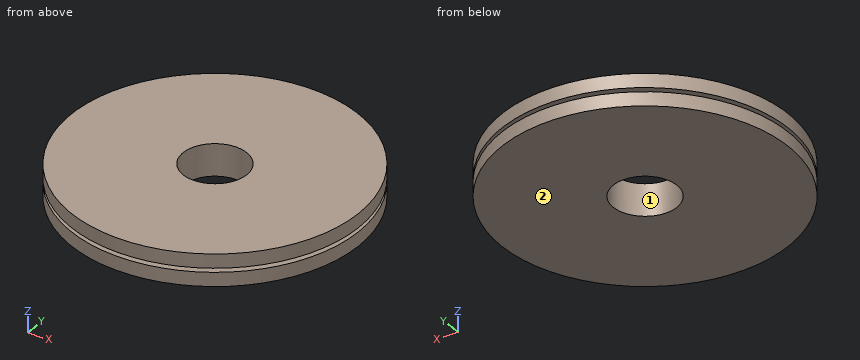
```python
from build123d import *

# Parameters (mm, degrees)
SKETCH1_R           = 57.15
SKETCH1_R_2         = 12.7
BOSS_EXTRUDE1_DEPTH = 12.7
SKETCH3_R           = 57.15
SKETCH3_R_2         = 53.975
CUT_EXTRUDE1_DEPTH  = 0.8001


with BuildPart() as part:
    # Sketch1 → Boss-Extrude1 (new body)
    with BuildSketch(Plane.XY):
        Circle(SKETCH1_R)
        Circle(SKETCH1_R_2, mode=Mode.SUBTRACT)
    extrude(amount=BOSS_EXTRUDE1_DEPTH)

    # Sketch3 → Cut-Extrude1 (cut, symmetric)
    with BuildSketch(Plane(origin=(0, 0, 6.35), x_dir=(-1, 0, 0), z_dir=(0, 0, -1))):
        Circle(SKETCH3_R)
        Circle(SKETCH3_R_2, mode=Mode.SUBTRACT)
    extrude(amount=CUT_EXTRUDE1_DEPTH, both=True, mode=Mode.SUBTRACT)


solid = part.part
```
The listing builds one solid part. Answer for the finished solid, in the listing's coordinates (mm). Face numbers are marked on the shaded views. Round coordinates to 2 decimals unless told otherwise and drop trailing zeros. Loops run counter-clockwise (first coordinate to the right, second up) from the corner with the lowest first, then second, coordinate; pieces in that order, holes last.
Q1. Section A-A, the plane x = 0 is taken. Determine the outline of the cut face in (y, z) (3 decimals), then the cut area to 3 significant figures.
Q2. Section C-C, the plane z = 3.25 is taken. Determine the outline of the cut face in (x, y), then the cut area to 3 significant figures.
Q3. For a pull along Y with two mould halves and no side action, classify the marked faces 1 and 2 as released by +Y, released by -Y, zero draft, split by the parting line, or undercut.
Q4. Section D-D, the plane y = 15 is taken. Determine the outline of the cut face in (x, z), then the cut area to 3 significant figures.
Q5. Given pin 1 Ø4 at (y, z) = (-38, 7.5) entering from +X; pin 2 Ø1 at (y, z) = (-12.5, 6) entering from +X; pin 3 Ø3 at (y, z) = (-32, 3.5) entering from +X; pin 4 Ø3 at (x, y) = (-37, 35) entering from -Z, each flat-ended and moving along its own axis, determine where each tip first touches the part or whether it passes through.
Q6. Find the intervals of material crossed by line 1 (Y direction, x = 0, z = 9); line 2 (X direction, y = 11.5, z = 7.25); line 3 (Y direction, x = -6, z = 9), in increasing order.
Completed:
1. outline: (-57.15, 0) - (-12.7, 0) - (-12.7, 12.7) - (-57.15, 12.7) - (-57.15, 7.15) - (-53.975, 7.15) - (-53.975, 5.55) - (-57.15, 5.55) - close; (12.7, 0) - (57.15, 0) - (57.15, 5.55) - (53.975, 5.55) - (53.975, 7.15) - (57.15, 7.15) - (57.15, 12.7) - (12.7, 12.7) - close
1. area: 1,120 mm2
2. outline: circle Ø114.3 at (0, 0); hole circle Ø25.4 at (0, 0)
2. area: 9,750 mm2
3. face 1: undercut
3. face 2: zero draft
4. outline: (-55.15, 0) - (55.15, 0) - (55.15, 5.55) - (51.85, 5.55) - (51.85, 7.15) - (55.15, 7.15) - (55.15, 12.7) - (-55.15, 12.7) - (-55.15, 7.15) - (-51.85, 7.15) - (-51.85, 5.55) - (-55.15, 5.55) - close
4. area: 1,390 mm2
5. pin 1: stops at x = 44.39
5. pin 2: stops at x = 55.81
5. pin 3: stops at x = 48.33
5. pin 4: stops at z = 0
6. line 1: y = -57.15 to -12.7, 12.7 to 57.15
6. line 2: x = -55.98 to -5.39, 5.39 to 55.98
6. line 3: y = -56.83 to -11.19, 11.19 to 56.83
